Can you work these out from the model? Positions are in its coordinate system, mm. Face numbers are marked on the shaded views. A direction names the side the tool comes from. Round coordinates to 2 decimals unless told otherwise and drop trailing zeros. Order: outer loops, then holes, each group sorted by start corner. A loop starts at its lowest first (then second) coordinate and runs counter-clockwise, first axis right, second up.
Q1. Will these pins go through, and if not, where does the flat tip stop? P1, Ø5, axis at x = 7, y = 5, coming from the +Z side; P2, Ø1.4, axis at x = 21.5, z = 2, coming from the -Y side; P3, Ø3, axis at x = -20, y = 0.5, coming from the +Z side; P4, Ø2, axis at y = 3.5, z = 4.5, coming from the +X side.
Q2. If we section it at D-D (x = 15): Please give me the cut outline in (y, z).
Q3. If I drill on line 1 (Y direction, x = -23, z = -0.6); line 2 (X direction, y = 1, z = 0.25); line 3 (Z direction, x = -7.5, y = 4), over which ranges is the centre line in solid material (lowest first)?
Q4. If we section it at B-B (y = -7): Please give me the cut outline in (x, z), plus the area to 3 significant figures.
Q5. If we section it at C-C (x = -16): Please give me the cut outline in (y, z), plus the area to 3 significant figures.
Q6. If we section it at A-A (z = -0.5): Please give me the cut outline in (x, y), plus the area to 3 significant figures.
Q7. For the marked faces 1, 2, 3 and 4, which set-ups out of +Z, -Z, +X, -X, +Y, -Y let a thin tool reach every point of the face, with its end or its side?
from build123d import *

# Parameters (mm, degrees)
F4_R     = 1.25
F4_W     = 18.1
F4_H     = 10
F4_W_2   = 8
F4_H_2   = 6
F4_W_3   = 5.6
F4_H_3   = 7.8
F5_DEPTH = 1.7
F6_DEPTH = 5.56
F7_DEPTH = 3.05
F8_DEPTH = 2.71


with BuildPart() as f5:
    # F4 (on Top) → F5 (new body)
    with BuildSketch(Plane.XY):
        with BuildLine():
            Line((23, 11.5), (-23, 11.5))
            ThreePointArc((-23, 11.5), (-24.767766953, 10.767766953), (-25.5, 9))
            Line((-25.5, 9), (-25.5, 5))
            Line((-25.5, 5), (-7.4, 5))
            Line((-7.4, 5), (-7.4, -5))
            Line((-7.4, -5), (-25.5, -5))
            Line((-25.5, -5), (-25.5, -9))
            ThreePointArc((-25.5, -9), (-24.767766953, -10.767766953), (-23, -11.5))
            Line((-23, -11.5), (11, -11.5))
            Line((11, -11.5), (11, -5.5))
            Line((11, -5.5), (19, -5.5))
            Line((19, -5.5), (19, -11.5))
            Line((19, -11.5), (23, -11.5))
            ThreePointArc((23, -11.5), (24.767766953, -10.767766953), (25.5, -9))
            Line((25.5, -9), (25.5, -3.9))
            Line((25.5, -3.9), (19.9, -3.9))
            Line((19.9, -3.9), (19.9, 3.9))
            Line((19.9, 3.9), (25.5, 3.9))
            Line((25.5, 3.9), (25.5, 9))
            ThreePointArc((25.5, 9), (24.767766953, 10.767766953), (23, 11.5))
        make_face()
        with Locations((-23, -9)):
            Circle(F4_R, mode=Mode.SUBTRACT)
        with Locations((23, -9)):
            Circle(F4_R, mode=Mode.SUBTRACT)
        with Locations((-23, 9)):
            Circle(F4_R, mode=Mode.SUBTRACT)
        with Locations((23, 9)):
            Circle(F4_R, mode=Mode.SUBTRACT)
        with Locations((-16.45, 0)):
            Rectangle(F4_W, F4_H)
        with Locations((15, -8.5)):
            Rectangle(F4_W_2, F4_H_2)
        with Locations((22.7, 0)):
            Rectangle(F4_W_3, F4_H_3)
    extrude(amount=-F5_DEPTH)

    # F4 (on Top) → F6 (join)
    with BuildSketch(Plane.XY):
        with Locations((15, -8.5)):
            Rectangle(F4_W_2, F4_H_2)
    extrude(amount=F6_DEPTH)

    # F4 (on Top) → F7 (join)
    with BuildSketch(Plane.XY):
        with Locations((-16.45, 0)):
            Rectangle(F4_W, F4_H)
    extrude(amount=F7_DEPTH)

    # F4 (on Top) → F8 (join)
    with BuildSketch(Plane.XY):
        with Locations((22.7, 0)):
            Rectangle(F4_W_3, F4_H_3)
    extrude(amount=F8_DEPTH)


solid = f5.part
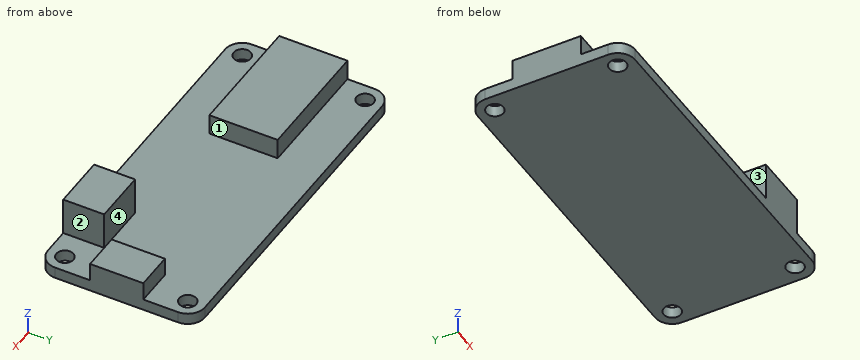
Solution:
1. P1: stops at z = 0
1. P2: stops at y = -3.9
1. P3: stops at z = 3.05
1. P4: passes through
2. outline: (-11.5, -1.7) - (11.5, -1.7) - (11.5, 0) - (-5.5, 0) - (-5.5, 5.56) - (-11.5, 5.56) - close
3. line 1: y = -11.5 to -10.25, -7.75 to 7.75, 10.25 to 11.5
3. line 2: x = -25.5 to -7.4, 19.9 to 25.5
3. line 3: z = -1.7 to 3.05
4. outline: (-25.5, -1.7) - (25.5, -1.7) - (25.5, 0) - (19, 0) - (19, 5.56) - (11, 5.56) - (11, 0) - (-25.5, 0) - close
4. area: 131 mm2
5. outline: (-11.5, -1.7) - (11.5, -1.7) - (11.5, 0) - (5, 0) - (5, 3.05) - (-5, 3.05) - (-5, 0) - (-11.5, 0) - close
5. area: 69.6 mm2
6. outline: (-25.5, -9) arc R2.5 ccw to (-23, -11.5) - (23, -11.5) arc R2.5 ccw to (25.5, -9) - (25.5, 9) arc R2.5 ccw to (23, 11.5) - (-23, 11.5) arc R2.5 ccw to (-25.5, 9) - close; hole circle Ø2.5 at (-23, -9); hole circle Ø2.5 at (-23, 9); hole circle Ø2.5 at (23, -9); hole circle Ø2.5 at (23, 9)
6. area: 1,150 mm2
7. face 1: +Z, +Y, -Y
7. face 2: +Z, +X, +Y, -Y
7. face 3: +Z, -X, +Y, -Y
7. face 4: +Z, +X, -X, +Y
